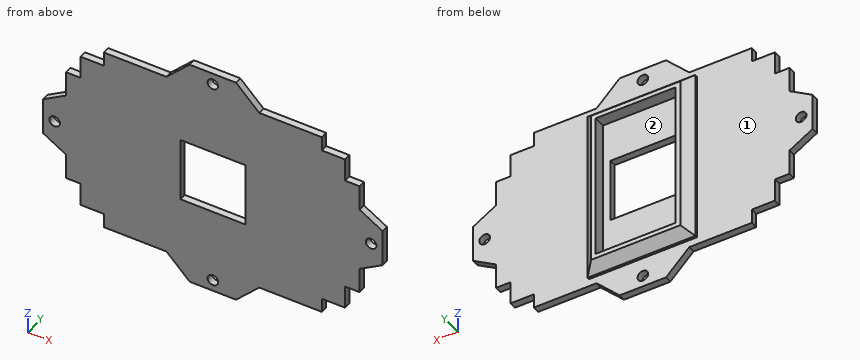
```python
from build123d import *

# Parameters (mm, degrees)
SKETCH_1_R      = 2.3
SKETCH_1_W      = 28
SKETCH_1_H      = 28
EXTRUDE_1_DEPTH = 3
SKETCH_2_W      = 46.5
SKETCH_2_H      = 76
SKETCH_2_W_2    = 34.5
SKETCH_2_H_2    = 64
EXTRUDE_2_DEPTH = 5
CHAMFER_1_SIZE  = 4


with BuildPart() as part:
    # Эскиз1 → Бобышка-Вытянуть1 (new body)
    with BuildSketch(Plane(origin=(0, 89.195974268, 0), x_dir=(1, 0, 0), z_dir=(0, 1, 0))):
        Polygon((44.808980694, -48.273129836), (54.808980694, -38.273129836), (74.808980694, -38.273129836), (84.808980694, -48.273129836), (111.808980694, -48.273129836), (111.808980694, -54.523129836), (121.808980694, -54.523129836), (121.808980694, -64.523129836), (128.058980694, -64.523129836), (128.058980694, -75.523129836), (138.058980694, -81.523129836), (138.058980694, -97.523129836), (128.058980694, -103.523129836), (128.058980694, -114.523129836), (121.808980694, -114.523129836), (121.808980694, -124.523129836), (111.808980694, -124.523129836), (111.808980694, -130.773129836), (84.808980694, -130.773129836), (74.808980694, -140.773129836), (54.808980694, -140.773129836), (44.808980694, -130.773129836), (17.808980694, -130.773129836), (17.808980694, -124.523129836), (7.808980694, -124.523129836), (7.808980694, -114.523129836), (1.558980694, -114.523129836), (1.558980694, -103.523129836), (-8.441019306, -97.523129836), (-8.441019306, -81.523129836), (1.558980694, -75.523129836), (1.558980694, -64.523129836), (7.808980694, -64.523129836), (7.808980694, -54.523129836), (17.808980694, -54.523129836), (17.808980694, -48.273129836), align=None)
        with Locations(Location((-3.441019306, -89.187817333, 0), (0, 0, 180))):
            Circle(SKETCH_1_R, mode=Mode.SUBTRACT)
        with Locations(Location((64.808980694, -43.273129836, 0), (0, 0, 180))):
            Circle(SKETCH_1_R, mode=Mode.SUBTRACT)
        with Locations(Location((133.058980694, -89.523129836, 0), (0, 0, 180))):
            Circle(SKETCH_1_R, mode=Mode.SUBTRACT)
        with Locations(Location((64.808980694, -135.773129836, 0), (0, 0, 180))):
            Circle(SKETCH_1_R, mode=Mode.SUBTRACT)
        with Locations((64.808980694, -89.523129836)):
            Rectangle(SKETCH_1_W, SKETCH_1_H, mode=Mode.SUBTRACT)
    extrude(amount=EXTRUDE_1_DEPTH)

    # Эскиз2 → Бобышка-Вытянуть2 (add)
    with BuildSketch(Plane(origin=(0, 92.195974268, 0), x_dir=(1, 0, 0), z_dir=(0, 1, 0))):
        with Locations((64.808980694, -89.523129836)):
            Rectangle(SKETCH_2_W, SKETCH_2_H)
        with Locations((64.808980694, -89.523129836)):
            Rectangle(SKETCH_2_W_2, SKETCH_2_H_2, mode=Mode.SUBTRACT)
    extrude(amount=EXTRUDE_2_DEPTH)

    # Фаска1
    chamfer_1_edges = [part.edges().sort_by_distance(p)[0] for p in [
        (41.558980694, 97.195974268, 89.523129836),
        (64.808980694, 97.195974268, 127.523129836),
        (88.058980694, 97.195974268, 89.523129836),
        (64.808980694, 97.195974268, 51.523129836),
    ]]
    chamfer(chamfer_1_edges, length=CHAMFER_1_SIZE)


solid = part.part
```
Can you work these out from the model? Positions are in its coordinate system, mm. Face numbers are marked on the shaded views. Round coordinates to 2 decimals unless told otherwise and drop trailing zeros. Loops run counter-clockwise (first coordinate to the right, second up) from the corner with the lowest first, then second, coordinate; pieces in that order, holes last. Notation, with made-up numbers: M -24.5,13 L -10.5,13 A14 ccw -10.5,34 Z; hole C -13.75,-2.75 d9. An arc over 180 degrees is marked long. Answer in a Markdown table with one row per item.
1. If we section it at A-A, the plane x = 60.5: Please give me the cut outline in (y, z), plus the area to 4 significant figures.
Established:
| item | result |
|---|---|
| outline | M 89.2,38.27 L 92.2,38.27 L 92.2,51.52 L 93.2,51.52 L 97.2,55.52 L 97.2,57.52 L 92.2,57.52 L 92.2,75.52 L 89.2,75.52 Z; M 89.2,103.52 L 92.2,103.52 L 92.2,121.52 L 97.2,121.52 L 97.2,123.52 L 93.2,127.52 L 92.2,127.52 L 92.2,140.77 L 89.2,140.77 Z |
| area | 267.5 mm² |
2. If we section it at C-C, the plane z = 109: Please give me the cut outline in (x, y), plus the area to 4 significant figures.
Established:
| item | result |
|---|---|
| outline | M 1.56,89.2 L 128.06,89.2 L 128.06,92.2 L 88.06,92.2 L 88.06,93.2 L 84.06,97.2 L 82.06,97.2 L 82.06,92.2 L 47.56,92.2 L 47.56,97.2 L 45.56,97.2 L 41.56,93.2 L 41.56,92.2 L 1.56,92.2 Z |
| area | 423.5 mm² |
3. I'm going to push flat-ended pins straight in: pin 1 Ø2.5 at (y, z) = (91, 128) entering from +X; pin 2 Ø2.5 at (y, z) = (90, 119.5) entering from +X; pin 3 Ø4 at (x, y) = (53.5, 94) entering from +Z; pin 4 Ø3.5 at (x, z) = (64.81, 43.27) entering from +Y. Where does each tip first touch, or does it pass through?
Established:
| item | result |
|---|---|
| pin 1 | x = 111.81 |
| pin 2 | x = 121.81 |
| pin 3 | z = 140.33 |
| pin 4 | through |
4. If we section it at D-D, the plane x = 80.5: Please give me the cut outline in (y, z).
Established:
| item | result |
|---|---|
| outline | M 89.2,43.96 L 92.2,43.96 L 92.2,51.52 L 93.2,51.52 L 97.2,55.52 L 97.2,57.52 L 92.2,57.52 L 92.2,121.52 L 97.2,121.52 L 97.2,123.52 L 93.2,127.52 L 92.2,127.52 L 92.2,135.08 L 89.2,135.08 Z |
5. If we section it at B-B, the plane z = 78: Please give me the cut outline in (x, y), plus the area to 3 significant figures.
Established:
| item | result |
|---|---|
| outline | M -2.57,89.2 L 50.81,89.2 L 50.81,92.2 L 47.56,92.2 L 47.56,97.2 L 45.56,97.2 L 41.56,93.2 L 41.56,92.2 L -2.57,92.2 Z; M 78.81,89.2 L 132.19,89.2 L 132.19,92.2 L 88.06,92.2 L 88.06,93.2 L 84.06,97.2 L 82.06,97.2 L 82.06,92.2 L 78.81,92.2 Z |
| area | 364 mm² |
6. Thinking about a two-plate mould opening in Z: for the marked faces 1 and 2, which applies, pulls with the +Z half, pulls with the -Z half, needs draft (parallel to the pull), parting line crosses it, or undercut?
Established:
| item | result |
|---|---|
| face 1 | needs draft |
| face 2 | undercut |
7. Please list where these lines run through material, in increasing order: line 1 (X direction, y = 92, z = 88); line 2 (X direction, y = 91.25, z = 70); line 3 (Y direction, x = 90, z = 129.5). Write a range as from..to.
Established:
| item | result |
|---|---|
| line 1 | -8.44..-5.41, -1.47..50.81, 78.81..131.34, 134.78..138.06 |
| line 2 | 1.56..128.06 |
| line 3 | 89.2..92.2 |
